```python
from build123d import *

# Parameters (mm, degrees)
SKETCH1_R           = 1.75
BOSS_EXTRUDE1_DEPTH = 2
BOSS_EXTRUDE2_START = 2
SKETCH1_3_R         = 1.75
BOSS_EXTRUDE2_DEPTH = 12.5


with BuildPart() as part:
    # Sketch1 → Boss-Extrude1 (new body)
    with BuildSketch(Plane.XY):
        Polygon((-23.65, 5.5), (-23.65, -5.5), (-11.6, -5.5), (-11.6, -1.5), (-16.15, -1.5), (-16.15, 1.5), (-11.6, 1.5), (-11.6, 5.5), align=None)
        with Locations((-19.9, 0)):
            Circle(SKETCH1_R, mode=Mode.SUBTRACT)
        Polygon((-11.6, 1.5), (-11.6, 5.5), (11.6, 5.5), (11.6, 1.5), (16.15, 1.5), (16.15, -1.5), (11.6, -1.5), (11.6, -5.5), (-11.6, -5.5), (-11.6, -1.5), (-16.15, -1.5), (-16.15, 1.5), align=None)
        Polygon((23.65, -5.5), (11.6, -5.5), (11.6, -1.5), (16.15, -1.5), (16.15, 1.5), (11.6, 1.5), (11.6, 5.5), (23.65, 5.5), align=None)
        with Locations((19.9, 0)):
            Circle(SKETCH1_R, mode=Mode.SUBTRACT)
    extrude(amount=BOSS_EXTRUDE1_DEPTH)

    # Sketch1<3> → Boss-Extrude2 (add)
    with BuildSketch(Plane.XY.offset(BOSS_EXTRUDE2_START)):
        Polygon((-23.65, 5.5), (-23.65, -5.5), (-11.6, -5.5), (-11.6, -1.5), (-16.15, -1.5), (-16.15, 1.5), (-11.6, 1.5), (-11.6, 5.5), align=None)
        with Locations((-19.9, 0)):
            Circle(SKETCH1_3_R, mode=Mode.SUBTRACT)
        Polygon((23.65, -5.5), (11.6, -5.5), (11.6, -1.5), (16.15, -1.5), (16.15, 1.5), (11.6, 1.5), (11.6, 5.5), (23.65, 5.5), align=None)
        with Locations((19.9, 0)):
            Circle(SKETCH1_3_R, mode=Mode.SUBTRACT)
    extrude(amount=BOSS_EXTRUDE2_DEPTH)


solid = part.part
```
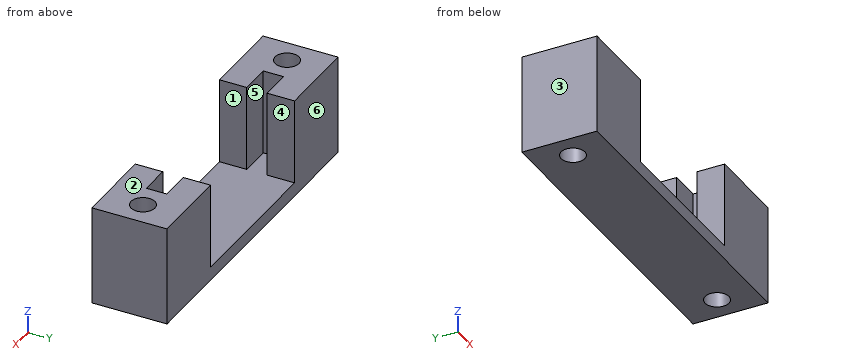
Could you check a few things on this model? Use its own coordinates, in mm. Face numbers are marked on the shaded views. A direction names the side the tool comes from. Round coordinates to 2 decimals unless told otherwise and drop trailing zeros. Loops run counter-clockwise (first coordinate to the right, second up) from the corner with the lowest first, then second, coordinate; pieces in that order, holes last. Notation, with made-up numbers: (45, 77) - (73, 77) arc R25 ccw to (73, 108) - close; hole circle Ø9 at (-38, 89.5). An arc over 180 degrees is marked (long way). Answer as CSV lines item,"result".
1. I want a section at A-A on z = 13. List the corners of the cut face in (x, y) for me.
Filled in:
outline,"(-23.65, -5.5) - (-11.6, -5.5) - (-11.6, -1.5) - (-16.15, -1.5) - (-16.15, 1.5) - (-11.6, 1.5) - (-11.6, 5.5) - (-23.65, 5.5) - close; (11.6, -5.5) - (23.65, -5.5) - (23.65, 5.5) - (11.6, 5.5) - (11.6, 1.5) - (16.15, 1.5) - (16.15, -1.5) - (11.6, -1.5) - close; hole circle Ø3.5 at (-19.9, 0); hole circle Ø3.5 at (19.9, 0)"
2. I want a section at D-D on z = 1.25. List the corners of the cut face in (x, y) for me, then the cut area to 3 significant figures.
Filled in:
outline,"(-23.65, -5.5) - (23.65, -5.5) - (23.65, 5.5) - (-23.65, 5.5) - close; hole circle Ø3.5 at (-19.9, 0); hole circle Ø3.5 at (19.9, 0)"
area,"501 mm^2"
3. On a 3-axis mill with a long thin cutter (end or side, diameter ignored), from which of +Z, -Z, +X, -X, +Y, -Y can I reach the whole of each face in a straight line? I mean the marked faces 4, 5 and 6. Say none if no direction works.
Filled in:
face 4,"+Z, +Y, -Y"
face 5,"+Z"
face 6,"+Z, -Z, +X, -X, +Y"
4. We'd pull the mould along X, two halves only. Please class the marked faces 1, 2 and 3: +X half, -X half, draft (parallel to the pull), parting line (faces both ways), or undercut.
Filled in:
face 1,"undercut"
face 2,"draft"
face 3,"-X half"
5. Please list where these lines run through material, in increasing order: line 1 along X through (y, z) = (-1, 13.5); line 2 along X through (y, z) = (2.25, 12.25); line 3 along Y through (x, z) = (-13, 13.25). Write a range as [from, to].
Filled in:
line 1,"x = [-23.65, -21.34], [-18.46, -16.15], [16.15, 18.46], [21.34, 23.65]"
line 2,"x = [-23.65, -11.6], [11.6, 23.65]"
line 3,"y = [-5.5, -1.5], [1.5, 5.5]"
6. I want a section at B-B on x = 19.9. List the corners of the cut face in (y, z) for me.
Filled in:
outline,"(-5.5, 0) - (-1.75, 0) - (-1.75, 14.5) - (-5.5, 14.5) - close; (1.75, 0) - (5.5, 0) - (5.5, 14.5) - (1.75, 14.5) - close"
7. I want a section at C-C on y = 0. List the corners of the cut face in (x, z) for me.
Filled in:
outline,"(-23.65, 0) - (-21.65, 0) - (-21.65, 14.5) - (-23.65, 14.5) - close; (-18.15, 0) - (18.15, 0) - (18.15, 14.5) - (16.15, 14.5) - (16.15, 2) - (-16.15, 2) - (-16.15, 14.5) - (-18.15, 14.5) - close; (21.65, 0) - (23.65, 0) - (23.65, 14.5) - (21.65, 14.5) - close"
8. For pin 1 Ø3 at (x, y) = (19.9, 0) entering from -Z; pin 2 Ø5 at (x, y) = (8, -3.5) entering from +Z, each with a flat end and sliding along its axis, tell me the tip position at first contact or that it passes through.
Filled in:
pin 1,"passes through"
pin 2,"stops at z = 2"
